Geometry: final body of the model. Coordinates: model frame, mm. A direction names the side the tool comes from. Coordinates: 2 decimals unless noted, no trailing zeros. Loops run counter-clockwise (first coordinate to the right, second up) from the corner with the lowest first, then second, coordinate; pieces in that order, holes last. Notation, with made-up numbers: M -29.75,-24 L 21.25,-24 A5 cw 21.25,-15 Z; hole C 76,84.25 d5. An arc over 180 degrees is marked long. Write item = value, one per line. Start each with the question number.
Autodesk Fusion 360 part; units mm, degrees
sketch "Sketch1" plane through (0, 0, 0) normal (0, 0, 1) x (1, 0, 0)
  line L0 (6.5, 14.8388) -> (6.5, -14.8388)
  line L1 (-6.5, -14.8388) -> (-6.5, 14.8388)
  line L2 (-6.5, 16.2) -> (6.5, -16.2) construction
  line L3 (6.5, 16.2) -> (-6.5, -16.2) construction
  arc A0 (-6.5, -14.8388) -> (6.5, -14.8388) centre (0, 0) ccw
  arc A1 (6.5, 14.8388) -> (-6.5, 14.8388) centre (0, 0) ccw
  line L4 (0, 0) -> (0, 6) construction
  circle A2 centre (0, -0.3) radius 2.5
  arc A3 (-0.0402, 0.1001) -> (0.0402, 0.1001) centre (0, 6) ccw
  arc A4 (2.3387, 0.5833) -> (-2.3387, 0.5833) centre (0, 6) ccw
  line L5 (0, 0) -> (0, -13.2) construction
  line L6 (0, -13.2) -> (6.5, -13.2)
  line L7 (0, -13.2) -> (-6.5, -13.2)
  line L8 (0, 16.2) -> (0, 12.2) construction
  line L9 (0, 12.2) -> (6.5, 12.2)
  line L10 (0, 12.2) -> (-6.5, 12.2)
  dimension "d1" = 32.4
  dimension "d2" = 13
  dimension "d3" = 32.4
  dimension "d4" = 6
  dimension "d5" = 11.8
  dimension "d6" = 5
  dimension "d9" = 13.2
  dimension "d10" = 4
extrude "Extrude1" add sketch "Sketch1" along normal blind 3
extrude "Extrude2" add sketch "Sketch1" against normal blind 1.5 contours L0 L1 A1 L9 L10 | L0 L1 A0 L6 L7
extrude "Extrude3" add 1 faces at (4.4187, -4.6534, 3) along direction (0, 0, 1) blind 1
Item 1: Section query A-A (x = 0). Return the cut outline in (y, z).
Item 2: First-contact query: pin 1 (4 mm diameter, centred on x = -0.5, y = -10, fed in from -Z); pin 2 (1.5 mm diameter, centred on x = 4.5, z = 1.5, fed in from +Y); pin 3 (1.5 mm diameter, centred on x = 4.5, z = -0.5, fed in from -Y). Flat tips, straight axial feed; report the tip coordinate or a pass-through.
Item 3: Section query D-D (x = -4.25). Return the cut outline in (y, z).
Item 4: Pull-direction query (Y, two-part tool) for faces 3 (the flat face through (0, 14, -1.5)), 4 (the cylindrical face through (-0.226, 11.896, 1.972)), 5 (the flat face through (0, 12.2, -1)), 6 (the cylindrical face through (-0.1, 16.2, 1.2)); classes: released by +Y, released by -Y, zero draft, split by the parting line, or undercut.
Item 5: Section query C-C (z = 1.65). Return the cut outline in (x, y), plus the area to 3 significant figures.
Item 6: Line query: line 1 (X direction, y = 6, z = 2.65); line 2 (X direction, y = -0.3, z = 1); line 3 (Z direction, x = 0, y = -4). Output: solid intervals per line, ascending. Write a range as from..to.
Item 7: Reachability of faces 1 (the cylindrical face through (0.1, -16.2, 1.2)), 2 (the flat face through (0, -13.2, -1)) from +Z, -Z, +X, -X, +Y, -Y: full face, straight path, thin tool, end or side. Return the list, or none.
Item 8: Section query B-B (y = 6). Return the cut outline in (x, z).
Verdict:
q1.outline = M -16.2,-1.5 L -13.2,-1.5 L -13.2,0 L -2.8,0 L -2.8,4 L -16.2,4 Z; M 11.9,0 L 12.2,0 L 12.2,-1.5 L 16.2,-1.5 L 16.2,4 L 11.9,4 Z
q2.pin_1 = 0
q2.pin_2 = 15.76
q2.pin_3 = -15.76
q3.outline = M -15.63,-1.5 L -13.2,-1.5 L -13.2,0 L 1.91,0 L 1.91,4 L -15.63,4 Z; M 10.09,0 L 12.2,0 L 12.2,-1.5 L 15.63,-1.5 L 15.63,4 L 10.09,4 Z
q4.face_3 = zero draft
q4.face_4 = undercut
q4.face_5 = undercut
q4.face_6 = released by +Y
q5.outline = M -6.5,-14.84 A16.2 ccw 6.5,-14.84 L 6.5,14.84 A16.2 ccw -6.5,14.84 Z; hole M -2.34,0.58 A2.5 ccw long 2.34,0.58 A5.9 ccw long Z
q5.area = 288 mm2
q6.line_1 = -6.5..-5.9, 5.9..6.5
q6.line_2 = -6.5..-2.5, 2.5..6.5
q6.line_3 = 0..4
q7.face_1 = +Z, -Z, -Y
q7.face_2 = -Z, +X, -X
q8.outline = M -6.5,0 L -5.9,0 L -5.9,4 L -6.5,4 Z; M 5.9,0 L 6.5,0 L 6.5,4 L 5.9,4 Z
